CAD build for the part. Positions are in the model's coordinates, mm. Face numbers are marked on the shaded views. A direction names the side the tool comes from. Round coordinates to 2 decimals unless told otherwise and drop trailing zeros. Loops run counter-clockwise (first coordinate to the right, second up) from the corner with the lowest first, then second, coordinate; pieces in that order, holes last. Notation, with made-up numbers: (-0.75, 14.5) - (15.25, 14.5) arc R31 ccw to (15.25, 43.5) - close; hole circle Ø2 at (40.5, 40). An arc over 180 degrees is marked (long way). Use one line per item in the form item = value.
from build123d import *

# Parameters (mm, degrees)
SKETCH029_W             = 42.3
SKETCH029_H             = 164.206055
PAD013_DEPTH            = 4
SKETCH030_W             = 42.3
SKETCH030_H             = 7
PAD014_DEPTH            = 42.3
SKETCH125_W             = 2
SKETCH125_H             = 35.8216107414
PAD049_DEPTH            = 42.3
SKETCH126_R             = 1.7
SKETCH126_R_2           = 10.9177905076
POCKET019_DEPTH         = 7
SKETCH127_R             = 1.7
SKETCH127_R_2           = 11.1
POCKET020_DEPTH         = 7
POCKET021_DEPTH         = 45
SKETCH129_R             = 11
POCKET022_DEPTH         = 7
SKETCH133_R             = 1.7
POCKET026_DEPTH         = 5
BODY025_PITCH_ANGLE     = 90
BODY025_PLACEMENT_ANGLE = -90


with BuildPart() as part:
    # Sketch029 → Pad013 (new body)
    with BuildSketch(Plane.YZ):
        with Locations((0, 4.8969725)):
            Rectangle(SKETCH029_W, SKETCH029_H)
    extrude(amount=PAD013_DEPTH)

    # Sketch030 (on Face6 of Pad013) → Pad014 (join)
    with BuildSketch(Plane.YZ.offset(4)):
        with Locations((0, 40.6783892586)):
            Rectangle(SKETCH030_W, SKETCH030_H)
        with Locations((0, 83.5)):
            Rectangle(SKETCH030_W, SKETCH030_H)
        with Locations((0, -73.706055)):
            Rectangle(SKETCH030_W, SKETCH030_H)
    extrude(amount=PAD014_DEPTH)

    # Sketch125 → Pad049 (join)
    with BuildSketch(Plane.YZ.offset(4)):
        with Locations((-20.15, 62.0891946293)):
            Rectangle(SKETCH125_W, SKETCH125_H)
        with Locations((20.15, 62.0891946293)):
            Rectangle(SKETCH125_W, SKETCH125_H)
    extrude(amount=PAD049_DEPTH)

    # Sketch126 (on Face20 of Pad049) → Pocket019 (cut)
    with BuildSketch(Plane.YX.offset(-37.1783892586)):
        with Locations((-15.5, 40.65)):
            Circle(SKETCH126_R)
        with Locations((15.5, 40.65)):
            Circle(SKETCH126_R)
        with Locations((15.5, 9.65)):
            Circle(SKETCH126_R)
        with Locations((-15.5, 9.65)):
            Circle(SKETCH126_R)
        with Locations((0, 25.15)):
            Circle(SKETCH126_R_2)
    extrude(amount=-POCKET019_DEPTH, mode=Mode.SUBTRACT)

    # Sketch127 (on Face24 of Pocket019) → Pocket020 (cut)
    with BuildSketch(Plane.YX.offset(-80)):
        with Locations((-15.5, 40.65)):
            Circle(SKETCH127_R)
        with Locations((15.5, 40.65)):
            Circle(SKETCH127_R)
        with Locations((15.5, 9.65)):
            Circle(SKETCH127_R)
        with Locations((-15.5, 9.65)):
            Circle(SKETCH127_R)
        with Locations((0, 25.15)):
            Circle(SKETCH127_R_2)
    extrude(amount=-POCKET020_DEPTH, mode=Mode.SUBTRACT)

    # Sketch128 (on Face14 of Pocket020) → Pocket021 (cut)
    with BuildSketch(Plane.ZX.offset(21.15)):
        with BuildLine():
            Line((55.6372167606, 40.749451), (68.417488, 40.749451))
            ThreePointArc((78.417488, 30.749451), (75.4885558119, 37.8205188119), (68.417488, 40.749451))
            Line((78.417488, 30.749451), (78.417488, 17.9691797606))
            ThreePointArc((68.417488, 7.9691797606), (75.4885558119, 10.8981119487), (78.417488, 17.9691797606))
            Line((68.417488, 7.9691797606), (55.6372167606, 7.9691797606))
            ThreePointArc((45.6372167606, 17.9691797606), (48.5661489487, 10.8981119487), (55.6372167606, 7.9691797606))
            Line((45.6372167606, 17.9691797606), (45.6372167606, 30.749451))
            ThreePointArc((55.6372167606, 40.749451), (48.5661489487, 37.8205188119), (45.6372167606, 30.749451))
        make_face()
    extrude(amount=-POCKET021_DEPTH, mode=Mode.SUBTRACT)

    # Sketch129 (on Face30 of Pocket021) → Pocket022 (cut)
    with BuildSketch(Plane(origin=(0, 0, -70.206055), x_dir=(0, -1, 0), z_dir=(0, 0, 1))):
        with Locations((0, 25.15)):
            Circle(SKETCH129_R)
    extrude(amount=-POCKET022_DEPTH, mode=Mode.SUBTRACT)

    # Sketch133 (on Face10 of Pocket022) → Pocket026 (cut)
    with BuildSketch(Plane.YZ.offset(4)):
        with Locations((-14.6419561845, 74.184478)):
            Circle(SKETCH133_R)
        with Locations((14.6419561845, 74.184478)):
            Circle(SKETCH133_R)
        with Locations((14.6419561845, -60.815522)):
            Circle(SKETCH133_R)
        with Locations((-14.6419561845, -60.815522)):
            Circle(SKETCH133_R)
    extrude(amount=-POCKET026_DEPTH, mode=Mode.SUBTRACT)


with BuildPart() as part_1:
    # Body025 pitch: moved
    add(part.part.rotate(Axis((0, 0, 0), (0, 1, 0)), BODY025_PITCH_ANGLE))


with BuildPart() as part_2:
    # Body025 placement: moved
    add(part_1.part.moved(Location((68, -1.5, 23))).rotate(Axis((68, -1.5, 23), (0, 0, 1)), BODY025_PLACEMENT_ANGLE))


solid = part_2.part
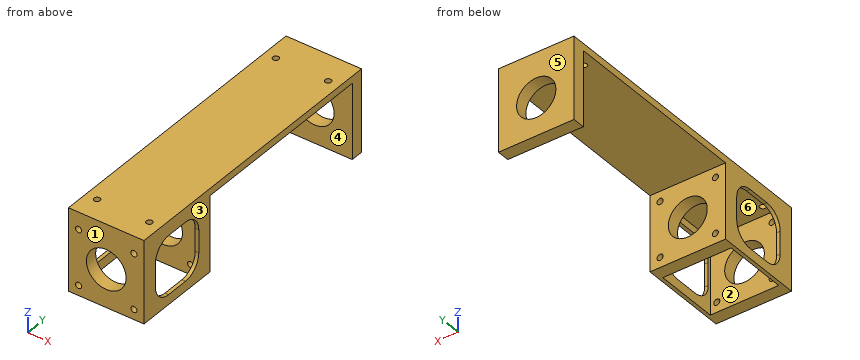
1) Flat gauge pins, fed straight in: pin 1 (1 mm diameter, centred on x = 60, y = -48, fed in from -Z); pin 2 (2.5 mm diameter, centred on x = 82.64, y = 59.32, fed in from +Z); pin 3 (2.5 mm diameter, centred on x = 83.5, z = 13.35, fed in from -Y). Where does each tip first touch, or does it go through?
Report:
pin_1 = 19
pin_2 = through
pin_3 = 68.71
2) Two-plate mould, pull along X, no slides. Class the marked faces 1, 2 and 3: +X half, -X half, draft (parallel to the pull), parting line (faces both ways), or undercut.
Report:
face_1 = draft
face_2 = undercut
face_3 = +X half
3) Slice it at C-C (y = 10.5). Write the cut outline in (x, z), plus the area to 3 significant figures.
Report:
outline = (46.85, 19) - (89.15, 19) - (89.15, 23) - (46.85, 23) - close
area = 169 mm^2
4) Slice it at B-B (z = -2.15). State how many separate pieces and enclosed holes the cut face has, plus the area to 3 significant figures.
Report:
separate_pieces = 6
enclosed_holes = 0
area = 438 mm^2
5) Drill centre lines: probe 1 along Y at (x, z) = (83.5, 5); probe 2 along Z at (x, y) = (83.5, -43.75); probe 3 along X at (y, z) = (-80, -16.5). Where is each one in solid material? Low to high.
Report:
probe_1 = -88.5 to -81.5, -45.68 to -38.68, 68.71 to 75.71
probe_2 = -23.3 to -19.35, -15.95 to 11.65, 15.05 to 23
probe_3 = 46.85 to 48.85, 87.15 to 89.15
6) Slice it at A-A (x = 68). Write the cut outline in (y, z), plus the area to 3 significant figures.
Report:
outline = (-88.5, -23.3) - (-81.5, -23.3) - (-81.5, -13.25) - (-88.5, -13.25) - close; (-88.5, 8.95) - (-81.5, 8.95) - (-81.5, 19) - (-45.68, 19) - (-45.68, 8.77) - (-38.68, 8.77) - (-38.68, 19) - (68.71, 19) - (68.71, 8.85) - (75.71, 8.85) - (75.71, 23) - (-88.5, 23) - close; (-45.68, -23.3) - (-38.68, -23.3) - (-38.68, -13.07) - (-45.68, -13.07) - close; (68.71, -23.3) - (75.71, -23.3) - (75.71, -13.15) - (68.71, -13.15) - close
area = 1,080 mm^2
7) Tool access for the marked faces 4, 5 and 6: list every direction of +Z, -Z, +X, -X, +Y, -Y with a clear straight run to the whole face (end or side of a thin tool).
Report:
face_4 = -Z, +X, -X
face_5 = +Z, -Z, +X, -X, +Y
face_6 = -Z
